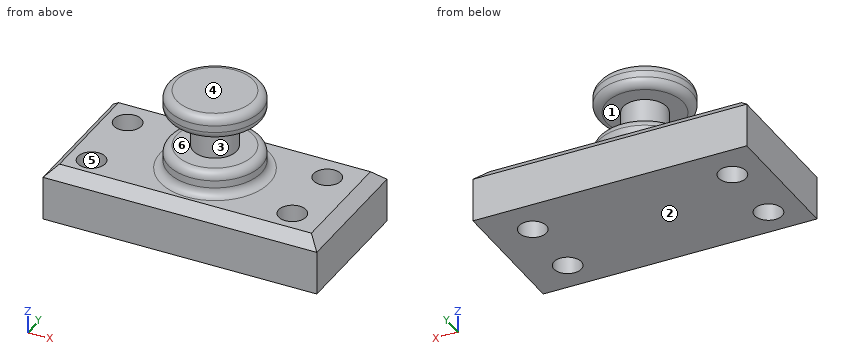
```python
from build123d import *

# Parameters (mm, degrees)
F0_W     = 127
F0_H     = 63.5
F1_DEPTH = 25.4
F3_D     = 12.7
F4_W     = 21.5339493006
F4_H     = 37.8580782562
F6_W     = 15.2821568772
F6_H     = 15.9768015146
F8_R     = 3.81
F9_SIZE  = 5.08


with BuildPart() as f1:
    # F0 (on Top) → F1 (new body)
    with BuildSketch(Plane.XY):
        Rectangle(F0_W, F0_H)
    extrude(amount=F1_DEPTH)

    # F3 (through all)
    with Locations(Plane(origin=(0, 0, 0), x_dir=(1, 0, 0), z_dir=(0, 0, -1))):
        with Locations((-48.0844858662, -14.7022493572), (-48.0844858662, 17.8973527858), (44.45, 16.7003627867), (44.5604218255, -14.7022493572)):
            Hole(F3_D / 2)

    # F4 (on Front) → F5 (revolve)
    with BuildSketch(Plane.XZ):
        with Locations((-10.7669746503, 44.3290391281)):
            Rectangle(F4_W, F4_H)
    revolve(axis=Axis((0, 0, 44.3290391281), (0, 0, 1)))

    # F6 (on Front) → F7 (revolve, cut)
    with BuildSketch(Plane.XZ):
        with Locations((-17.7134093828, 44.4571860135)):
            Rectangle(F6_W, F6_H)
    revolve(axis=Axis((0, 0, 63.2580782562), (0, 0, -1)), mode=Mode.SUBTRACT)

    # F8
    f8_edges = [f1.edges().sort_by_distance(p)[0] for p in [
        (21.533949, 0, 63.258078),
        (21.533949, 0, 36.468785),
        (21.533949, 0, 25.4),
        (21.533949, 0, 52.445587),
    ]]
    fillet(f8_edges, radius=F8_R)

    # F9
    f9_edges = [f1.edges().sort_by_distance(p)[0] for p in [
        (0, 31.75, 25.4),
        (-63.5, 0, 25.4),
        (0, -31.75, 25.4),
        (63.5, 0, 25.4),
    ]]
    chamfer(f9_edges, length=F9_SIZE)


solid = f1.part
```
Design review of the part built by this model. Coordinates are the model's own, in mm. Face numbers are marked on the shaded views. A direction names the side the tool comes from. Coordinates: 2 decimals unless noted, no trailing zeros. Order: outer loops, then holes, each group sorted by start corner. A loop starts at its lowest first (then second) coordinate and runs counter-clockwise, first axis right, second up. Notation, with made-up numbers: (35.5, 55.5) - (53.5, 55.5) arc R29 cw to (53.5, 91.5) - close; hole circle Ø8 at (62.25, 51.5). An arc over 180 degrees is marked (long way). One line per question, with ' | ' between items.
Q1. Consider section A-A, the plane x = 0. Give the boundary of the cut face in (y, z).
Answer key:
outline: (-31.75, 0) - (31.75, 0) - (31.75, 20.32) - (26.67, 25.4) - (25.34, 25.4) arc R3.81 cw to (21.53, 29.21) - (21.53, 32.66) arc R3.81 ccw to (17.72, 36.47) - (10.07, 36.47) - (10.07, 52.45) - (17.72, 52.45) arc R3.81 ccw to (21.53, 56.26) - (21.53, 59.45) arc R3.81 ccw to (17.72, 63.26) - (-17.72, 63.26) arc R3.81 ccw to (-21.53, 59.45) - (-21.53, 56.26) arc R3.81 ccw to (-17.72, 52.45) - (-10.07, 52.45) - (-10.07, 36.47) - (-17.72, 36.47) arc R3.81 ccw to (-21.53, 32.66) - (-21.53, 29.21) arc R3.81 cw to (-25.34, 25.4) - (-26.67, 25.4) - (-31.75, 20.32) - close
Q2. To check wall thickness, follow line 1 along Y through (x, z) = (44.45, 17); line 2 along Z through (x, y) = (-6.5, -10); line 3 along Z through (x, y) = (-3, -25.5). State the ranges of each line that lie inside material, in increasing order.
Answer key:
line 1: y = -31.75 to -23.05, -10.35 to 8.35, 21.05 to 31.75 | line 2: z = 0 to 36.47, 52.45 to 63.26 | line 3: z = 0 to 25.4
Q3. For the marked faces 1 and 2, list the 3-axis set-ups (+Z, -Z, +X, -X, +Y, -Y) from which the entire face can be reached by the end or side of a thin tool; tool diameter is ignored.
Answer key:
face 1: none | face 2: -Z, +X, -X, +Y, -Y
Q4. Consider section C-C, the plane x = -43.5. Give the boundary of the cut face in (y, z), then the cut area to 3 significant figures.
Answer key:
outline: (-31.75, 0) - (-22.29, 0) - (-22.29, 25.4) - (-26.67, 25.4) - (-31.75, 20.32) - close; (-13.5, 0) - (10.31, 0) - (10.31, 25.4) - (-13.5, 25.4) - close; (19.1, 0) - (31.75, 0) - (31.75, 20.32) - (26.67, 25.4) - (19.1, 25.4) - close | area: 1,140 mm2
Q5. Clearance check with flat-ended pins moving along their axes: pin 1 Ø1.5 at (y, z) = (-13, 33) entering from -X; pin 2 Ø7.5 at (x, y) = (44.56, 14.7) entering from -Z (3 decimals); pin 3 Ø6 at (y, z) = (22.5, 32) entering from -X; pin 4 Ø3 at (y, z) = (-10, 52.5) entering from +X. State where each tip first meets the part, or that it passes through.
Answer key:
pin 1: stops at x = -17.7 | pin 2: passes through | pin 3: stops at x = -9.14 | pin 4: stops at x = 18.45
Q6. Consider section D-D, the plane y = 0. Give the boundary of the cut face in (x, z), then the cut area to 3 significant figures.
Answer key:
outline: (-63.5, 0) - (63.5, 0) - (63.5, 20.32) - (58.42, 25.4) - (25.34, 25.4) arc R3.81 cw to (21.53, 29.21) - (21.53, 32.66) arc R3.81 ccw to (17.72, 36.47) - (10.07, 36.47) - (10.07, 52.45) - (17.72, 52.45) arc R3.81 ccw to (21.53, 56.26) - (21.53, 59.45) arc R3.81 ccw to (17.72, 63.26) - (-17.72, 63.26) arc R3.81 ccw to (-21.53, 59.45) - (-21.53, 56.26) arc R3.81 ccw to (-17.72, 52.45) - (-10.07, 52.45) - (-10.07, 36.47) - (-17.72, 36.47) arc R3.81 ccw to (-21.53, 32.66) - (-21.53, 29.21) arc R3.81 cw to (-25.34, 25.4) - (-58.42, 25.4) - (-63.5, 20.32) - close | area: 4,450 mm2
Q7. Consider section B-B, the plane z = 22. Give the boundary of the cut face in (x, y), then the cut area to 3 significant figures.
Answer key:
outline: (-61.82, -30.07) - (61.82, -30.07) - (61.82, 30.07) - (-61.82, 30.07) - close; hole circle Ø12.7 at (-48.08, -17.9); hole circle Ø12.7 at (-48.08, 14.7); hole circle Ø12.7 at (44.45, -16.7); hole circle Ø12.7 at (44.56, 14.7) | area: 6,930 mm2
Q8. The part is to be moulded in two halves that separate along Z. For the marked faces 3, 4, 5 and 6, say which applies: +Z half, -Z half, draft (parallel to the pull), parting line (faces both ways), or undercut.
Answer key:
face 3: undercut | face 4: +Z half | face 5: draft | face 6: undercut
